Design review of the part built by this model. Coordinates are the model's own, in mm. Face numbers are marked on the shaded views. A direction names the side the tool comes from. Give positions to 0.01 mm unless a question says otherwise; leave off trailing zeros. Write each loop counter-clockwise with the first axis right and the second up, starting at its lowest first coordinate (ties: lowest second). Pieces come first, ordered by that corner, then holes. Notation, with made-up numbers: M -24.75,24 L 15.25,24 A32 cw 15.25,51 Z; hole C 1,70 d3. An arc over 180 degrees is marked long. Answer in a Markdown table with one row per item.
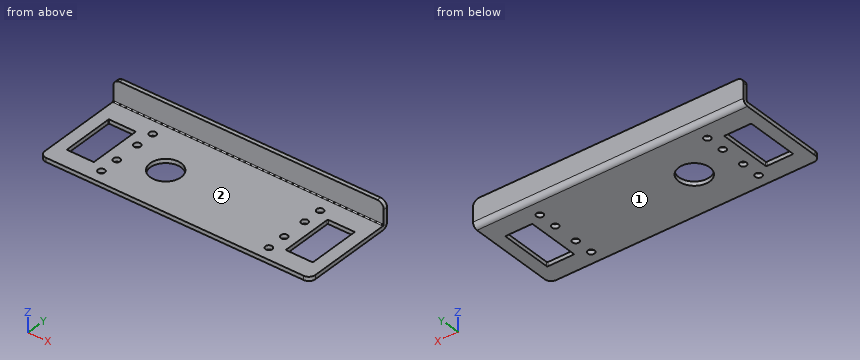
```python
from build123d import *

# Parameters (mm, degrees)
SKETCH1_W                    = 210
SKETCH1_H                    = 75
SKETCH1_R                    = 11.9875
SKETCH1_W_2                  = 21
SKETCH1_H_2                  = 41
BASE_FLANGE1_DEPTH           = 3.175
EDGE_FLANGE1_STRIP_W         = 14.1732
EDGE_FLANGE1_STRIP_H         = 3.175
EDGE_FLANGE1_STRIP_CUT_DEPTH = 210
EDGE_FLANGE1_DEPTH           = 210
M5_CLEARANCE_HOLE1_D         = 5.3
FILLET1_R                    = 5
FILLET2_R                    = 0.5


# Sheet-metal steps are written as plain solids
with BuildPart() as part:
    # Sketch1 → Base-Flange1 (new body)
    with BuildSketch(Plane.XY):
        with Locations((35, 2.5)):
            Rectangle(SKETCH1_W, SKETCH1_H)
        Circle(SKETCH1_R, mode=Mode.SUBTRACT)
        with Locations((-50, 0)):
            Rectangle(SKETCH1_W_2, SKETCH1_H_2, mode=Mode.SUBTRACT)
        with Locations((120, 0)):
            Rectangle(SKETCH1_W_2, SKETCH1_H_2, mode=Mode.SUBTRACT)
    extrude(amount=-BASE_FLANGE1_DEPTH)

    # Edge-Flange1 strip (across the edge) → Edge-Flange1 strip cut (cut)
    with BuildSketch(Plane(origin=(140, 40, 0), x_dir=(0, -1, 0), z_dir=(-1, 0, 0))):
        with Locations((-3.175, -1.5875)):
            Rectangle(EDGE_FLANGE1_STRIP_W, EDGE_FLANGE1_STRIP_H)
    extrude(amount=EDGE_FLANGE1_STRIP_CUT_DEPTH, mode=Mode.SUBTRACT)

    # Edge-Flange1 section (across the edge) → Edge-Flange1 (add)
    with BuildSketch(Plane(origin=(140, 40, 0), x_dir=(0, -1, 0), z_dir=(-1, 0, 0))):
        with BuildLine():
            Line((0, 0.7366), (0, 16.825))
            Line((0, 16.825), (3.175, 16.825))
            Line((3.175, 16.825), (3.175, 0.7366))
            ThreePointArc((3.175, 0.7366), (3.390745145, 0.215745145), (3.9116, 0))
            Line((3.9116, 0), (3.9116, -3.175))
            ThreePointArc((3.9116, -3.175), (1.145681115, -2.029318885), (0, 0.7366))
        make_face()
    extrude(amount=EDGE_FLANGE1_DEPTH)

    # M5 Clearance Hole1 (through all)
    with Locations(Plane(origin=(-30, 25, 0), x_dir=(1, 0, 0), z_dir=(0, 0, 1))):
        with Locations((0, 0), (0, -50), (130, -50), (130, 0), (0, -15), (0, -35), (130, -35), (130, -15)):
            Hole(M5_CLEARANCE_HOLE1_D / 2)

    # Fillet1
    fillet1_edges = [part.edges().sort_by_distance(p)[0] for p in [
        (140, 38.4125, 16.825),
        (-70, 38.4125, 16.825),
        (140, -35, -1.5875),
        (-70, -35, -1.5875),
    ]]
    fillet(fillet1_edges, radius=FILLET1_R)

    # Fillet2
    fillet2_edges = [part.edges().sort_by_distance(p)[0] for p in [
        (-60.5, -20.5, -1.5875),
        (-60.5, 20.5, -1.5875),
        (-39.5, 20.5, -1.5875),
        (-39.5, -20.5, -1.5875),
        (109.5, -20.5, -1.5875),
        (109.5, 20.5, -1.5875),
        (130.5, 20.5, -1.5875),
        (130.5, -20.5, -1.5875),
    ]]
    fillet(fillet2_edges, radius=FILLET2_R)


solid = part.part
```
1) Insertion check: P1, Ø3, axis at x = -45, y = 25, coming from the +Z side; P2, Ø8.5, axis at x = -30, y = -10, coming from the -Z side (3 decimals); P3, Ø4, axis at x = 65, z = 9.5, coming from the -Y side (3 decimals). Each pin has a flat end and moves straight along its axis. Give the tip position at first contact, or say it passes through.
Geometry says:
| item | result |
|---|---|
| P1 | z = 0 |
| P2 | z = -3.175 |
| P3 | y = 36.825 |
2) Add section C-C (x = -30). Write out the cut boundary in (y, z) (3 decimals).
Geometry says:
| item | result |
|---|---|
| outline | M -35,-3.175 L -27.65,-3.175 L -27.65,0 L -35,0 Z; M -22.35,-3.175 L -12.65,-3.175 L -12.65,0 L -22.35,0 Z; M -7.35,-3.175 L 7.35,-3.175 L 7.35,0 L -7.35,0 Z; M 12.65,-3.175 L 22.35,-3.175 L 22.35,0 L 12.65,0 Z; M 27.65,-3.175 L 36.088,-3.175 A3.912 ccw 40,0.737 L 40,16.825 L 36.825,16.825 L 36.825,0.737 A0.737 cw 36.088,0 L 27.65,0 Z |
3) Add section A-A (y = -15). Write out the cut boundary in (x, z) (3 decimals), and give its area (3 significant figures).
Geometry says:
| item | result |
|---|---|
| outline | M -70,-3.175 L -60.5,-3.175 L -60.5,0 L -70,0 Z; M -39.5,-3.175 L 109.5,-3.175 L 109.5,0 L -39.5,0 Z; M 130.5,-3.175 L 140,-3.175 L 140,0 L 130.5,0 Z |
| area | 533 mm^2 |
4) Add section B-B (x = 0). Write out the cut boundary in (y, z) (1 decimal).
Geometry says:
| item | result |
|---|---|
| outline | M -35,-3.2 L -12,-3.2 L -12,0 L -35,0 Z; M 12,-3.2 L 36.1,-3.2 A3.9 ccw 40,0.7 L 40,16.8 L 36.8,16.8 L 36.8,0.7 A0.7 cw 36.1,0 L 12,0 Z |
5) Add section D-D (x = 51). Write out the cut boundary in (y, z) (3 decimals), and give its area (3 significant figures).
Geometry says:
| item | result |
|---|---|
| outline | M -35,-3.175 L 36.088,-3.175 A3.912 ccw 40,0.737 L 40,16.825 L 36.825,16.825 L 36.825,0.737 A0.737 cw 36.088,0 L -35,0 Z |
| area | 288 mm^2 |
6) For the marked faces 1 and 2, list the 3-axis set-ups (+Z, -Z, +X, -X, +Y, -Y) from which the entire face can be reached by the end or side of a thin tool; tool diameter is ignored.
Geometry says:
| item | result |
|---|---|
| face 1 | -Z, +X, -X, +Y, -Y |
| face 2 | +Z, +X, -X, -Y |
7) To check wall thickness, follow probe 1 along Y at (x, z) = (100, -1.7); probe 2 along Y at (x, z) = (4, 8) (3 decimals); probe 3 along Z at (x, y) = (12.5, -25) (3 decimals). State the ranges of each line that lie inside material, in increasing order. Write a range as [from, to].
Geometry says:
| item | result |
|---|---|
| probe 1 | [-35, -27.65], [-22.35, -12.65], [-7.35, 7.35], [12.65, 22.35], [27.65, 39.15] |
| probe 2 | [36.825, 40] |
| probe 3 | [-3.175, 0] |
